Geometry: final body of the model. Coordinates: model frame, mm. Give positions to 0.01 mm unless a question says otherwise; leave off trailing zeros. Write each loop counter-clockwise with the first axis right and the second up, starting at its lowest first coordinate (ties: lowest second). Pieces come first, ordered by that corner, then holes. Notation, with made-up numbers: M 26.25,-6 L 83.25,-6 A7 ccw 83.25,5 Z; hole C 69,23 d11. An arc over 180 degrees is marked long. Answer as a JSON object with one key per item and string values.
Autodesk Inventor part; units mm, degrees
ref_plane "YZ Plane" through (0, 0, 0) normal (1, 0, 0) x (0, 1, 0)
ref_plane "XZ Plane" through (0, 0, 0) normal (0, 1, 0) x (-1, 0, 0)
ref_plane "XY Plane" through (0, 0, 0) normal (0, 0, 1) x (1, 0, 0)
sketch "Esboço1" plane through (0, 0, 0) normal (0, 0, 1) x (1, 0, 0)
  circle A0 centre (0, 0) radius 3.175
  line L0 (20.5, 0) -> (20.5, 7.6069)
  dimension "d1" = 6.35
revolve "Revolução1" add sketch "Esboço1" angle 180 about axis through (20.5, 0, 0) along (0, -1, 0)
sketch "Esboço2" plane through (0, 0, 0) normal (0, 0, 1) x (1, 0, 0)
  circle A0 centre (0, 0) radius 3.175
  circle A1 centre (41, 0) radius 3.175
  circle A2 centre (41, 0) radius 3.175
extrude "Extrusão1" add sketch "Esboço2" along normal blind 58
thread "Rosca1"
thread "Rosca2"
chamfer "Chanfro1" distance 0.5 angle 45 2 edges at (-3.175, 0, 58) (37.825, 0, 58)
properties part number "0070.1 - Abraçadeira U Vergalhão bitola 1 polegada 80mm rosca 1 quarto" material "Aço, carbono"
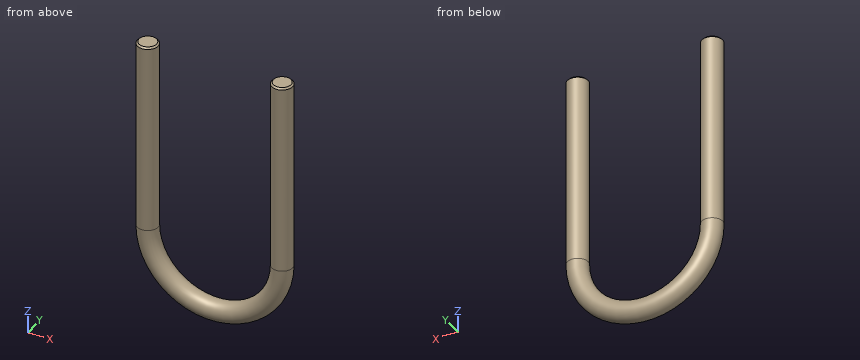
1) Cut plane A-A on y = 0. Return loops of the section in (x, z) (3 decimals), and give its area (3 significant figures).
Geometry check:
{"outline": "M -3.175,0 A23.675 ccw 44.175,0 L 44.175,57.5 L 43.675,58 L 38.325,58 L 37.825,57.5 L 37.825,0 A17.325 cw 3.175,0 L 3.175,57.5 L 2.675,58 L -2.675,58 L -3.175,57.5 Z", "area": "1,150 mm2"}
2) Cut plane B-B on z = 16.5. Return loops of the section in (x, y) (3 decimals), and give its area (3 significant figures).
Geometry check:
{"outline": "C 0,0 d6.35; C 41,0 d6.35", "area": "63.3 mm2"}
3) Line query: line 1 (X direction, y = 0.25, z = 20); line 2 (X direction, y = -1.5, z = -7.5); line 3 (Z direction, x = 13.5, y = 1.25). Output: solid intervals per line, ascending. Write a range as from..to.
Geometry check:
{"line 1": "x = -3.17..3.17, 37.83..44.17", "line 2": "x = -1.56..4.47, 36.53..42.56", "line 3": "z = -22.35..-16.13"}
4) Contact query for flat-ended pins moving along their axis: P1, Ø1, axis at x = 35.5, y = 0, coming from the +Z side; P2, Ø1.5, axis at y = 1, z = 30.5, coming from the -X side. Output: stop coordinate, or through.
Geometry check:
{"P1": "stops at z = -7.74", "P2": "stops at x = -3.17"}
